Here's how the part is built. I have some questions about the finished solid (model axes, mm). A direction names the side the tool comes from. Round coordinates to 2 decimals unless told otherwise and drop trailing zeros. Write each loop counter-clockwise with the first axis right and the second up, starting at its lowest first coordinate (ties: lowest second). Pieces come first, ordered by that corner, then holes. Notation, with made-up numbers: M 65,-7 L 108,-7 A24 cw 108,3 Z; hole C 35,-13.75 d9. An arc over 180 degrees is marked long. Use one line per item in the form item = value. Start each with the question number.
Q1. I want a section at D-D on z = 4. List the corners of the cut face in (x, y) for me, and give its area (3 significant figures).
Q2. For faces 4 (the face through (-10, -7, 13)), 5 (the face through (-0.14, -19.85, 9.85)), 6 (the face through (-11, -6, 1)), which set-ups out of +Z, -Z, +X, -X, +Y, -Y let a thin tool reach every point of the face, with its end or its side?
Q3. I'm going to push flat-ended pins straight in: pin 1 Ø2.5 at (x, y) = (5, 0) entering from -Z; pin 2 Ø6 at (x, y) = (19, -14) entering from -Z; pin 3 Ø4 at (x, y) = (19.5, -8) entering from +Z; pin 4 Ø1 at (x, z) = (6.5, 8.5) entering from -Y. Where does each tip first touch, or does it pass through?
Q4. I need wall thicknesses on line 1 along Y through (x, z) = (5, 2.4); line 2 along X through (y, z) = (-13.5, 3.25); line 3 along Y through (x, z) = (10, 1.75). Which ranges of each line are inside material? Lowest first, please. Write a range as from..to.
Q5. I want a section at C-C on y = -15. List the corners of the cut face in (x, z) for me.
Q6. I want a section at A-A on x = -5. List the corners of the cut face in (y, z) for me.
Q7. We'd pull the mould along Z, two halves only. Please class faces 1 (the face through (0, -6, 0)), 2 (the face through (2.5, -16, 7)), 3 (the face through (-0.14, -11.157, 12.178)): +Z half, -Z half, draft (parallel to the pull), parting line (faces both ways), or undercut.
Q8. I want a section at B-B on y = 0. List the corners of the cut face in (x, z) for me.
```python
from build123d import *

# Parameters (mm, degrees)
SKETCH_1_W          = 22
SKETCH_1_H          = 10
SKETCH_1_R          = 1.65
EXTRUDE_1_DEPTH     = 3
SKETCH_2_W          = 22
SKETCH_2_H          = 3
EXTRUDE_2_DEPTH     = 13
SKETCH_4_W          = 5
SKETCH_4_H          = 5
EXTRUDE_3_DEPTH     = 8
EXTRUDE_4_DEPTH     = 25
SKETCH_7_R          = 0.91
CUT_EXTRUDE_1_DEPTH = 30
SKETCH_8_W          = 20
SKETCH_8_H          = 8
CUT_EXTRUDE_2_DEPTH = 5


with BuildPart() as part:
    # 草图1 → 凸台-拉伸1 (new body)
    with BuildSketch(Plane.XY):
        Rectangle(SKETCH_1_W, SKETCH_1_H)
        with Locations((-5, 0)):
            Circle(SKETCH_1_R, mode=Mode.SUBTRACT)
        with Locations(Location((5, 0, 0), (0, 0, 180))):
            Circle(SKETCH_1_R, mode=Mode.SUBTRACT)
    extrude(amount=EXTRUDE_1_DEPTH)

    # 草图2 → 凸台-拉伸2 (add)
    with BuildSketch(Plane.XZ.offset(5)):
        with Locations((0, 1.5)):
            Rectangle(SKETCH_2_W, SKETCH_2_H)
    extrude(amount=EXTRUDE_2_DEPTH)

    # 草图4 → 凸台-拉伸3 (add)
    with BuildSketch(Plane.XY.offset(3)):
        with Locations((0, -15.5)):
            Rectangle(SKETCH_4_W, SKETCH_4_H)
    extrude(amount=EXTRUDE_3_DEPTH)

    # 草图6 → 凸台-拉伸4 (add, symmetric)
    with BuildSketch(Plane.ZY):
        Polygon((6.79883611, -27.315253784), (13.269312237, -3.167108126), (15.20116389, -3.684746216), (8.730687763, -27.832891874), align=None)
    extrude(amount=EXTRUDE_4_DEPTH, both=True)

    # 草图7 → 切除-拉伸1 (cut)
    with BuildSketch(Plane(origin=(0, -4.047122166, 15.104065547), x_dir=(1, 0, 0), z_dir=(0, -0.25881904510251497, 0.9659258262890699))):
        with Locations(Location((-21.41, -3.254840811, 0), (0, 0, 270))):
            Circle(SKETCH_7_R)
        with Locations(Location((21.41, -3.254840811, 0), (0, 0, 270))):
            Circle(SKETCH_7_R)
        with Locations(Location((21.41, -20.994840811, 0), (0, 0, 270))):
            Circle(SKETCH_7_R)
        with Locations(Location((-21.41, -20.994840811, 0), (0, 0, 270))):
            Circle(SKETCH_7_R)
    extrude(amount=-CUT_EXTRUDE_1_DEPTH, mode=Mode.SUBTRACT)

    # 草图8 → 切除-拉伸2 (cut)
    with BuildSketch(Plane(origin=(0, -4.047122166, 15.104065547), x_dir=(1, 0, 0), z_dir=(0, -0.25881904510251497, 0.9659258262890699))):
        with Locations((0, -3.624840811)):
            Rectangle(SKETCH_8_W, SKETCH_8_H)
        with Locations((0, -20.624840811)):
            Rectangle(SKETCH_8_W, SKETCH_8_H)
    extrude(amount=-CUT_EXTRUDE_2_DEPTH, mode=Mode.SUBTRACT)


solid = part.part
```
Reported:
q1.outline = M -2.5,-18 L 2.5,-18 L 2.5,-13 L -2.5,-13 Z
q1.area = 25.0 mm^2
q2.face_4 = +Z, +Y
q2.face_5 = -Z, -Y
q2.face_6 = -Z, -X, +Y, -Y
q3.pin_1 = through
q3.pin_2 = 9.56
q3.pin_3 = 14.58
q3.pin_4 = -19.62
q4.line_1 = -18..-1.65, 1.65..5
q4.line_2 = -2.5..2.5
q4.line_3 = -18..5
q5.outline = M -25,10.1 L -2.5,10.1 L -2.5,3 L -11,3 L -11,0 L 11,0 L 11,3 L 2.5,3 L 2.5,10.1 L 25,10.1 L 25,12.17 L -25,12.17 Z
q6.outline = M -20.11,10.8 L -19.59,8.87 L -10.89,11.2 L -11.41,13.13 Z; M -18,0 L -1.65,0 L -1.65,3 L -18,3 Z; M 1.65,0 L 5,0 L 5,3 L 1.65,3 Z
q7.face_1 = -Z half
q7.face_2 = undercut
q7.face_3 = +Z half
q8.outline = M -11,0 L -6.65,0 L -6.65,3 L -11,3 Z; M -3.35,0 L 3.35,0 L 3.35,3 L -3.35,3 Z; M 6.65,0 L 11,0 L 11,3 L 6.65,3 Z
